```python
from build123d import *

# Parameters (mm, degrees)
SKETCH_1_W          = 10
SKETCH_1_H          = 10
EXTRUDE_1_DEPTH     = 175
SKETCH_2_W          = 8
SKETCH_2_H          = 8
CUT_EXTRUDE_1_DEPTH = 351.071421284
SKETCH_3_R          = 1.6
CUT_EXTRUDE_2_DEPTH = 176.356779168
SKETCH_4_R          = 1.6
CUT_EXTRUDE_3_DEPTH = 176.356779168
SKETCH_5_R          = 1.6
CUT_EXTRUDE_4_DEPTH = 176.356779168


with BuildPart() as part:
    # Sketch 1 → Extrude 1 (new, symmetric)
    with BuildSketch(Plane(origin=(0, 0, 0), x_dir=(0, 0, -1), z_dir=(1, 0, 0))):
        Rectangle(SKETCH_1_W, SKETCH_1_H)
    extrude(amount=EXTRUDE_1_DEPTH, both=True)

    # Sketch 2 → Cut-Extrude 1 (cut, through all)
    with BuildSketch(Plane(origin=(175, 0, 0), x_dir=(0, 0, -1), z_dir=(1, 0, 0))):
        Rectangle(SKETCH_2_W, SKETCH_2_H)
    extrude(amount=-CUT_EXTRUDE_1_DEPTH, mode=Mode.SUBTRACT)

    # Sketch 3 → Cut-Extrude 2 (cut, through all)
    with BuildSketch(Plane(origin=(0, 5, 0), x_dir=(1, 0, 0), z_dir=(0, 1, 0))):
        with Locations(Location((-170, 0, 0), (0, 0, 270))):
            Circle(SKETCH_3_R)
        with Locations(Location((-155, 0, 0), (0, 0, 270))):
            Circle(SKETCH_3_R)
        with Locations(Location((170, 0, 0), (0, 0, 270))):
            Circle(SKETCH_3_R)
        with Locations(Location((155, 0, 0), (0, 0, 270))):
            Circle(SKETCH_3_R)
    extrude(amount=-CUT_EXTRUDE_2_DEPTH, mode=Mode.SUBTRACT)

    # Sketch 4 → Cut-Extrude 3 (cut, through all)
    with BuildSketch(Plane(origin=(0, 5, 0), x_dir=(1, 0, 0), z_dir=(0, 1, 0))):
        with Locations(Location((-75, 0, 0), (0, 0, 270))):
            Circle(SKETCH_4_R)
        with Locations(Location((-60, 0, 0), (0, 0, 270))):
            Circle(SKETCH_4_R)
        with Locations(Location((-45, 0, 0), (0, 0, 270))):
            Circle(SKETCH_4_R)
        with Locations(Location((45, 0, 0), (0, 0, 270))):
            Circle(SKETCH_4_R)
        with Locations(Location((60, 0, 0), (0, 0, 270))):
            Circle(SKETCH_4_R)
        with Locations(Location((75, 0, 0), (0, 0, 270))):
            Circle(SKETCH_4_R)
    extrude(amount=-CUT_EXTRUDE_3_DEPTH, mode=Mode.SUBTRACT)

    # Sketch 5 → Cut-Extrude 4 (cut, through all)
    with BuildSketch(Plane.XY.offset(5)):
        with Locations((-35, 0)):
            Circle(SKETCH_5_R)
        with Locations((35, 0)):
            Circle(SKETCH_5_R)
    extrude(amount=-CUT_EXTRUDE_4_DEPTH, mode=Mode.SUBTRACT)


solid = part.part
```
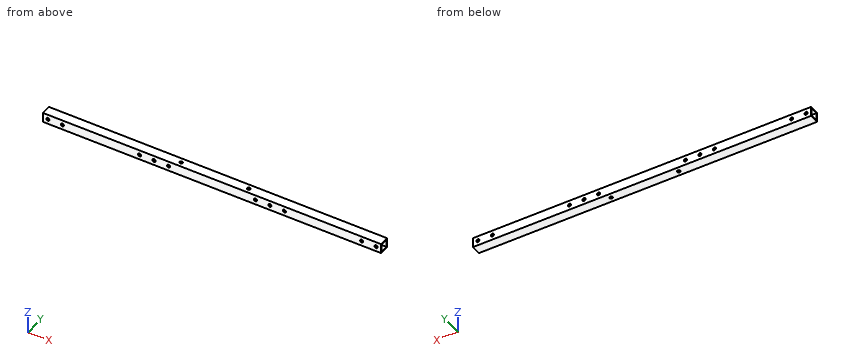
Geometry check sheet. Reference: the model listing, model coordinates, mm. Give positions to 0.01 mm unless a question says otherwise; leave off trailing zeros. Write each loop counter-clockwise with the first axis right and the second up, starting at its lowest first coordinate (ties: lowest second). Pieces come first, ordered by that corner, then holes. Notation, with made-up numbers: (-29.5, 17) - (-15.5, 17) arc R19 cw to (-15.5, 35) - close; hole circle Ø4 at (23, -31.75). An arc over 180 degrees is marked (long way). Use a Markdown table: item, result.
Q1. Section check B-B, the plane y = 0. Enter the section's corners in (x, z).
Computed:
| item | result |
|---|---|
| outline | (-175, -5) - (-36.6, -5) - (-36.6, -4) - (-175, -4) - close; (-175, 4) - (-36.6, 4) - (-36.6, 5) - (-175, 5) - close; (-33.4, -5) - (33.4, -5) - (33.4, -4) - (-33.4, -4) - close; (-33.4, 4) - (33.4, 4) - (33.4, 5) - (-33.4, 5) - close; (36.6, -5) - (175, -5) - (175, -4) - (36.6, -4) - close; (36.6, 4) - (175, 4) - (175, 5) - (36.6, 5) - close |
Q2. Go/stop test with flat-tipped pins: P1, Ø2.5, axis at x = -75, z = 0, coming from the -Y side; P2, Ø5, axis at x = 45, z = 0, coming from the +Y side. Record where each tip stops, or that it passes through.
Computed:
| item | result |
|---|---|
| P1 | passes through |
| P2 | stops at y = 5 |
Q3. Section check A-A, the plane x = 93. Enter the section's corners in (y, z), then the cut area to 3 significant figures.
Computed:
| item | result |
|---|---|
| outline | (-5, -5) - (5, -5) - (5, 5) - (-5, 5) - close; hole (-4, -4) - (4, -4) - (4, 4) - (-4, 4) - close |
| area | 36.0 mm² |
Q4. Section check C-C, the plane z = 0. Give the number of separate pieces and of enclosed holes in the cut face, then the cut area to 3 significant figures.
Computed:
| item | result |
|---|---|
| separate pieces | 22 |
| enclosed holes | 0 |
| area | 636 mm² |
Q5. Thickness scan on L1, parallel to Y at x = 5, z = 1; L2, parallel to Z at x = -154, y = 4.5. Record the ranges inside material, lowest first. Write a range as [from, to].
Computed:
| item | result |
|---|---|
| L1 | y = [-5, -4], [4, 5] |
| L2 | z = [-5, -1.25], [1.25, 5] |
